```python
from build123d import *

# Parameters (mm, degrees)
F1_DEPTH = 28.575
F3_DEPTH = 22.86
F5_DEPTH = 177.8
F6_R     = 1.27


with BuildPart() as f1:
    # F0 (on Right) → F1 (new body, symmetric)
    with BuildSketch(Plane.YZ):
        Polygon((-57.9421781003, 88.9), (-57.9421781003, 0), (-38.8921781003, 0), (-38.8921781003, 3.175), (-35.7171781003, 3.175), (-35.7171781003, 0), (97.6328218997, 0), (97.6328218997, 3.175), (100.8078218997, 3.175), (100.8078218997, 0), (119.8578218997, 0), align=None)
    extrude(amount=F1_DEPTH, both=True)

    # F2 (on face) → F3 (cut)
    with BuildSketch(Plane(origin=(0, 0, 0), x_dir=(1, 0, 0), z_dir=(0, 0, -1))):
        Polygon((11.43, 33.4499907649), (0, 33.4499907649), (-11.43, 33.4499907649), (-11.43, 10.5899907649), (0, 10.5899907649), (11.43, 10.5899907649), align=None)
    extrude(amount=-F3_DEPTH, mode=Mode.SUBTRACT)

    # F4 (on face) → F5 (intersect)
    with BuildSketch(Plane.XZ.offset(57.9421781003)):
        Polygon((-9.9975576818, 16.3837641232), (-28.575, 0), (28.575, 0), (9.9975576818, 16.3837641232), (0, 60.9972961555), align=None)
    extrude(amount=-F5_DEPTH, mode=Mode.INTERSECT)

    # F6
    f6_edges = [f1.edges().sort_by_distance(p)[0] for p in [
        (0, 119.857822, 0),
        (4.998779, 42.476762, 38.69053),
        (-4.998779, 42.476762, 38.69053),
        (19.286279, 103.474058, 8.191882),
        (-19.286279, 103.474058, 8.191882),
        (0, -30.039474, 60.997296),
        (9.997558, 38.250151, 16.383764),
        (28.575, 30.957822, 0),
        (28.575, -48.417178, 0),
        (28.575, 110.332822, 0),
        (-28.575, 110.332822, 0),
        (-28.575, 30.957822, 0),
        (-28.575, -48.417178, 0),
        (-9.997558, 38.250151, 16.383764),
        (-9.997558, -45.696084, 16.383764),
        (9.997558, -45.696084, 16.383764),
    ]]
    fillet(f6_edges, radius=F6_R)


solid = f1.part
```
Geometry check sheet. Reference: the model listing, model coordinates, mm. A direction names the side the tool comes from. Give positions to 0.01 mm unless a question says otherwise; leave off trailing zeros. Loops run counter-clockwise (first coordinate to the right, second up) from the corner with the lowest first, then second, coordinate; pieces in that order, holes last. Notation, with made-up numbers: M 52,-35 L 76,-35 A25 ccw 76,0 Z; hole C -34.75,-22.75 d7. An arc over 180 degrees is marked long. Write item = value, one per line.
(1) Material ranges on line 1 (Y direction, x = 12, z = 2.5); line 2 (Y direction, x = -4.5, z = 18); line 3 (Y direction, x = -1, z = 12), recorded low to high. Write a range as [from, to].
Answer below:
line_1 = [-57.94, -38.89], [-35.72, 97.63], [100.81, 114.86]
line_2 = [-57.94, -33.45], [-10.59, 83.86]
line_3 = [-57.94, -33.45], [-10.59, 95.86]
(2) Release check for a two-part mould opening along X. For faces 1 (the face through (0, -10.59, 11)), 2 (the face through (0, -33.45, 11)), 3 (the face through (6.597, -3.735, 31.558)), 4 (the face through (0, -22, 22.86)) record: released by +X, released by -X, zero draft, split by the parting line, or undercut.
Answer below:
face_1 = undercut
face_2 = undercut
face_3 = released by +X
face_4 = zero draft
(3) Sectioned sample at A-A, the plane y = -18. Record the cut outline in (x, z), plus the area to 3 significant figures.
Answer below:
outline = M -26.05,2.22 A1.27 ccw -25.21,0 L -11.43,0 L -11.43,15.12 Z; M -8.55,22.86 L 8.55,22.86 L 1.24,55.47 A1.27 ccw -1.24,55.47 Z; M 11.43,0 L 25.21,0 A1.27 ccw 26.05,2.22 L 11.43,15.12 Z
area = 576 mm2
(4) Gauge pin test, flat ends, axial feed: pin 1 Ø10 at (x, z) = (-7.5, 10.5) entering from +Y; pin 2 Ø13.5 at (x, y) = (-0.5, -26.5) entering from -Z; pin 3 Ø4.5 at (y, z) = (-20.5, 10.5) entering from -X. Record the tip position at first contact, or that the pin passes through.
Answer below:
pin_1 = 108.86
pin_2 = 22.86
pin_3 = -19.22
(5) Tool access check on faces 5 (the face through (0, -38.892, 2)), 6 (the face through (5.2, 46.2, 36.5)), 7 (the face through (-11.43, -22, 7)). Record the directions out of +Z, -Z, +X, -X, +Y, -Y that give a thin tool (end or side, any length) a straight path to the whole face; none if there is none.
Answer below:
face_5 = -Z, +X, -X
face_6 = +Z, +X, +Y
face_7 = +Z, -Z
